The listing builds one solid part. Answer for the finished solid, in the listing's coordinates (mm). Face numbers are marked on the shaded views. Round coordinates to 2 decimals unless told otherwise and drop trailing zeros. Write each loop counter-clockwise with the first axis right and the second up, starting at its lowest first coordinate (ties: lowest second). Pieces come first, ordered by that corner, then holes.
Item 1: Find section B-B on y = -11. Give the vertices of the cut face in (x, z), then the cut area to 3 significant figures.
Item 2: Find section C-C on x = 16. Give the vertices of the cut face in (y, z) (3 decimals).
Item 3: For a pull along Y with two mould halves and no side action, classify the marked faces 1, 2, 3 and 4 as +Y half, -Y half, draft (parallel to the pull), parting line (faces both ways), or undercut.
Item 4: Find section A-A on z = 18.65. Give the number of separate pieces and of enclosed holes in the cut face, then the cut area to 3 significant figures.
Item 5: Find the intervals of material crossed by probe 1 along Z at (x, y) = (16, -7); probe 2 along Y at (x, z) = (14.75, -13.5); probe 3 along Z at (x, y) = (16, 8.5), in increasing order.
Item 6: Find section D-D on z = -19. Give the vertices of the cut face in (x, y), then the cut area to 3 significant figures.
Item 7: Each of these flat-tipped pins is pushed along its axis until it touches: pin 1 (7 mm diameter, centred on x = 14, z = 19.5, fed in from -Y); pin 2 (6.5 mm diameter, centred on x = 5, z = 18.65, fed in from -Y); pin 3 (3.5 mm diameter, centred on x = 11.5, y = 1, fed in from +Z); pin 4 (1.9 mm diameter, centred on x = 5, z = 18.65, fed in from -Y). Where does it stop, or does it pass through?
```python
from build123d import *

# Parameters (mm, degrees)
F1_DEPTH       = 21
F3_W           = 6.55
F3_H           = 12.7
F4_DEPTH       = 21.001
F5_D           = 4.2
F5_DEPTH       = 14
F5_CBORE_D     = 8.25
F5_CBORE_DEPTH = 4
F5_TIP         = 1.2618073
F7_D           = 3.2
F7_DEPTH       = 20
F7_TIP         = 0.9613769904
F8_DEPTH       = 1


with BuildPart() as f1:
    # F0 (on Right) → F1 (new body)
    with BuildSketch(Plane.YZ):
        Polygon((-16, 25), (-16, -25), (-1, -25), (-1, -5), (1, -5), (1, -25), (16, -25), (16, 25), align=None)
    extrude(amount=F1_DEPTH)

    # F3 (on face) → F4 (cut, through all)
    with BuildSketch(Plane.YZ.offset(21)):
        with Locations((0, 18.65)):
            Rectangle(F3_W, F3_H)
    extrude(amount=-F4_DEPTH, mode=Mode.SUBTRACT)

    # F5
    with Locations(Plane.XZ.offset(16)):
        with Locations((5, 18.65), (16, 18.65)):
            CounterBoreHole(F5_D / 2, F5_CBORE_D / 2, F5_CBORE_DEPTH, depth=F5_DEPTH)
            with Locations((0, 0, -(F5_DEPTH + F5_TIP / 2))):  # 118° drill point
                Cone(0, F5_D / 2, F5_TIP, mode=Mode.SUBTRACT)

    # F7
    with Locations(Plane(origin=(0, 16, 0), x_dir=(-1, 0, 0), z_dir=(0, 1, 0))):
        with Locations((-16, 18.65), (-5, 18.65)):
            Hole(F7_D / 2, depth=F7_DEPTH)
            with Locations((0, 0, -(F7_DEPTH + F7_TIP / 2))):  # 118° drill point
                Cone(0, F7_D / 2, F7_TIP, mode=Mode.SUBTRACT)

    # F8 (add): faces of the model
    f8_faces = [f1.faces().sort_by_distance(p)[0] for p in [
        (10.5, -9.6375, 25),
        (10.5, 9.6375, 25),
    ]]
    extrude(f8_faces, amount=F8_DEPTH)


solid = f1.part
```
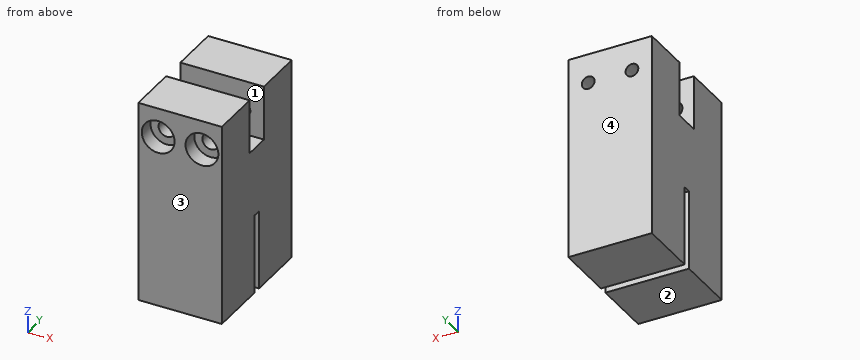
Check values:
1. outline: (0, -25) - (21, -25) - (21, 26) - (0, 26) - close; hole circle Ø4.2 at (5, 18.65); hole circle Ø4.2 at (16, 18.65)
1. area: 1,040 mm2
2. outline: (-16, -25) - (-1, -25) - (-1, -5) - (1, -5) - (1, -25) - (16, -25) - (16, 17.05) - (3.275, 17.05) - (3.275, 12.3) - (-3.275, 12.3) - (-3.275, 16.55) - (-12, 16.55) - (-12, 14.525) - (-16, 14.525) - close; (-16, 22.775) - (-12, 22.775) - (-12, 20.75) - (-3.275, 20.75) - (-3.275, 26) - (-16, 26) - close; (3.275, 20.25) - (16, 20.25) - (16, 26) - (3.275, 26) - close
3. face 1: undercut
3. face 2: draft
3. face 3: -Y half
3. face 4: +Y half
4. separate pieces: 6
4. enclosed holes: 0
4. area: 314 mm2
5. probe 1: z = -25 to 16.55, 20.75 to 26
5. probe 2: y = -16 to -1, 1 to 16
5. probe 3: z = -25 to 17.05, 20.25 to 26
6. outline: (0, -16) - (21, -16) - (21, -1) - (0, -1) - close; (0, 1) - (21, 1) - (21, 16) - (0, 16) - close
6. area: 630 mm2
7. pin 1: stops at y = -16
7. pin 2: stops at y = -12
7. pin 3: stops at z = 12.3
7. pin 4: passes through
